Answer from the drawing. Dimensions are ordinates in mm from the lowest x, y and z of the part. A direction names the side the tool comes from. Coordinates: 2 decimals unless noted, no trailing zeros. Write each loop counter-clockwise with the first axis right and the second up, starting at its lowest first coordinate (ties: lowest second). Pieces come first, ordered by that corner, then holes. Notation, with made-up numbers: (-4.5, -2) - (54.5, -2) arc R20 ccw to (54.5, 25) - close; hole circle Ø2 at (33.25, 31). An arc over 180 degrees is marked (long way). Return JSON: item names as keys, results as strings.
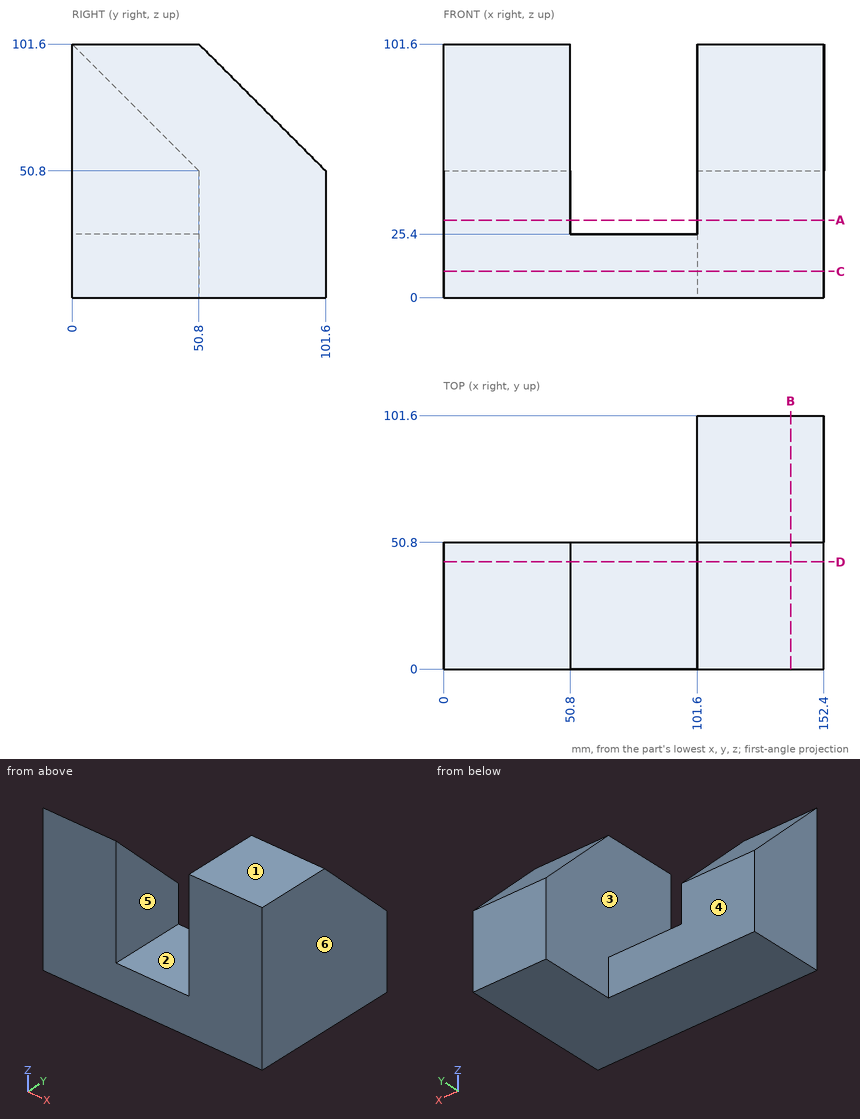
(1) Straight lines are drawn through the part: line 1 (X direction, y = 25.5, z = 63); line 2 (X direction, y = 72, z = 28.5); line 3 (Y direction, x = 92, z = 14). For each, find the intervals that lie inside material, in ascending order. Write a range as from..to.
Answer:
{"line 1": "0..50.8, 101.6..152.4", "line 2": "101.6..152.4", "line 3": "0..50.8"}
(2) A cutting plane is placed at D-D (y = 43). Determine the outline of the cut face in (x, z), and give its area (3 significant figures).
Answer:
{"outline": "(0, 0) - (152.4, 0) - (152.4, 101.6) - (101.6, 101.6) - (101.6, 25.4) - (50.8, 25.4) - (50.8, 58.6) - (0, 58.6) - close", "area": "9,430 mm²"}
(3) A cutting plane is placed at B-B (x = 139). Determine the outline of the cut face in (y, z), and give its area (3 significant figures).
Answer:
{"outline": "(0, 0) - (101.6, 0) - (101.6, 50.8) - (50.8, 101.6) - (0, 101.6) - close", "area": "9,030 mm²"}
(4) Determine the mould class of the marked faces 3, 4, 5 and 6 for opening direction X: +X half, -X half, draft (parallel to the pull), parting line (faces both ways), or undercut.
Answer:
{"face 3": "undercut", "face 4": "draft", "face 5": "undercut", "face 6": "+X half"}
(5) A cutting plane is placed at C-C (z = 10.5). Determine the outline of the cut face in (x, y), and give its area (3 significant figures).
Answer:
{"outline": "(0, 0) - (152.4, 0) - (152.4, 101.6) - (101.6, 101.6) - (101.6, 50.8) - (0, 50.8) - close", "area": "10,300 mm²"}
(6) Which of the six approach directions +Z, -Z, +X, -X, +Y, -Y give full straight-line access (tool end or side, diameter ignored) to the marked faces 1 and 2?
Answer:
{"face 1": "+Z, +X, -X, +Y, -Y", "face 2": "+Z, +Y, -Y"}
(7) A flat-ended cylindrical pin translates along its axis: P1, Ø1.5, axis at x = 96, y = 34, coming from the -Z side. Find the tip coordinate at first contact, or state that the pin passes through.
Answer:
{"P1": "z = 0"}
(8) A cutting plane is placed at A-A (z = 31). Determine the outline of the cut face in (x, y).
Answer:
{"outline": "(0, 0) - (50.8, 0) - (50.8, 50.8) - (0, 50.8) - close; (101.6, 0) - (152.4, 0) - (152.4, 101.6) - (101.6, 101.6) - close"}
